The model under review builds one solid part; all positions refer to its coordinate system, in mm. Face numbers are marked on the shaded views. A direction names the side the tool comes from. Round coordinates to 2 decimals unless told otherwise and drop trailing zeros. Write each loop counter-clockwise with the first axis right and the second up, starting at its lowest first coordinate (ties: lowest second). Pieces come first, ordered by that corner, then holes. Notation, with made-up numbers: (-12.5, -3.75) - (22.5, -3.75) arc R25 ccw to (22.5, 31.25) - close; hole circle Ø1 at (40, -26). An arc over 180 degrees is marked (long way). Return JSON: item names as keys, results as strings.
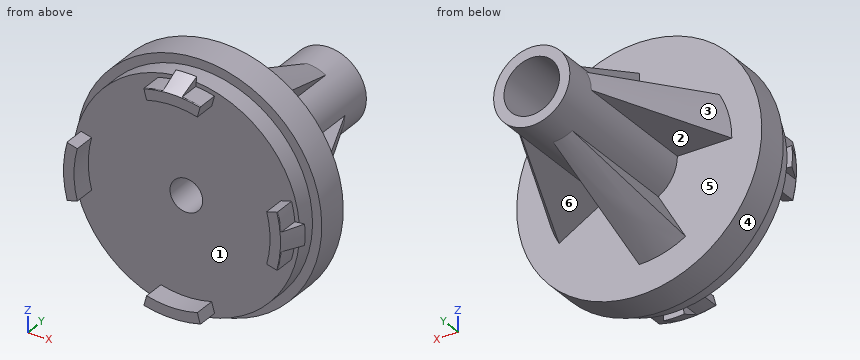
from build123d import *

# Parameters (mm, degrees)
SKETCH_1_R          = 10.4
EXTRUDE_1_DEPTH     = 1.8
SKETCH_2_R          = 11.25
EXTRUDE_2_DEPTH     = 3
SKETCH_3_R          = 3.5
SKETCH_3_R_2        = 2.55
EXTRUDE_3_DEPTH     = 15
SKETCH_3_4_R        = 1.5
CUT_EXTRUDE_2_DEPTH = 4.8
REVOLVE_3_ANGLE     = 30
REVOLVE_4_ANGLE     = 30
EXTRUDE_4_DEPTH     = 2


with BuildPart() as part:
    # 草图1 → 凸台-拉伸1 (new body)
    with BuildSketch(Plane(origin=(0, 0, 0), x_dir=(1, 0, 0), z_dir=(0, 1, 0))):
        with Locations(Location((0, 0, 0), (0, 0, 270))):
            Circle(SKETCH_1_R)
    extrude(amount=EXTRUDE_1_DEPTH)

    # 草图2 → 凸台-拉伸2 (add)
    with BuildSketch(Plane(origin=(0, 1.8, 0), x_dir=(1, 0, 0), z_dir=(0, 1, 0))):
        with Locations(Location((0, 0, 0), (0, 0, 270))):
            Circle(SKETCH_2_R)
    extrude(amount=EXTRUDE_2_DEPTH)

    # 草图3 → 凸台-拉伸3 (add)
    with BuildSketch(Plane(origin=(0, 4.8, 0), x_dir=(1, 0, 0), z_dir=(0, 1, 0))):
        with Locations(Location((0, 0, 0), (0, 0, 270))):
            Circle(SKETCH_3_R)
        with Locations(Location((0, 0, 0), (0, 0, 270))):
            Circle(SKETCH_3_R_2, mode=Mode.SUBTRACT)
    extrude(amount=EXTRUDE_3_DEPTH)

    # 草图3<4> → 切除-拉伸2 (cut)
    with BuildSketch(Plane(origin=(0, 4.8, 0), x_dir=(1, 0, 0), z_dir=(0, 1, 0))):
        with Locations(Location((0, 0, 0), (0, 0, 270))):
            Circle(SKETCH_3_4_R)
    extrude(amount=-CUT_EXTRUDE_2_DEPTH, mode=Mode.SUBTRACT)

    # 草图6 → 旋转3 (revolve)
    with BuildSketch(Plane(origin=(0, 0, 0), x_dir=(0, 0, -1), z_dir=(1, 0, 0))):
        Polygon((3.5, 4.8), (3.5, 16.8), (8.5, 4.8), align=None)
        Polygon((-8.5, 4.8), (-3.5, 4.8), (-3.5, 16.8), align=None)
    revolve(axis=Axis((0, 0, 0), (0, 1, 0)), revolution_arc=REVOLVE_3_ANGLE)

    # 草图9 → 旋转4 (revolve)
    with BuildSketch(Plane.XY):
        Polygon((3.5, 4.8), (8.5, 4.8), (3.5, 16.8), align=None)
        Polygon((-8.5, 4.8), (-3.5, 16.8), (-3.5, 4.8), align=None)
    revolve(axis=Axis((0, 0, 0), (0, 1, 0)), revolution_arc=REVOLVE_4_ANGLE)

    # 草图10 → 凸台-拉伸4 (add)
    with BuildSketch(Plane.XZ):
        with BuildLine():
            Line((9.961946981, -0.871557427), (10.858522209, -0.949997596))
            ThreePointArc((10.858522209, -0.949997596), (10.9, 0), (10.858522209, 0.949997596))
            Line((10.858522209, 0.949997596), (9.961946981, 0.871557427))
            ThreePointArc((9.961946981, 0.871557427), (9.84807753, 1.736481777), (9.659258263, 2.588190451))
            Line((9.659258263, 2.588190451), (8.693332437, 2.329371406))
            ThreePointArc((8.693332437, 2.329371406), (9, 0), (8.693332437, -2.329371406))
            Line((8.693332437, -2.329371406), (9.659258263, -2.588190451))
            ThreePointArc((9.659258263, -2.588190451), (9.84807753, -1.736481777), (9.961946981, -0.871557427))
        make_face()
        with BuildLine():
            Line((2.329371406, 8.693332437), (2.588190451, 9.659258263))
            ThreePointArc((2.588190451, 9.659258263), (1.736481777, 9.84807753), (0.871557427, 9.961946981))
            Line((0.871557427, 9.961946981), (0.949997596, 10.858522209))
            ThreePointArc((0.949997596, 10.858522209), (0, 10.9), (-0.949997596, 10.858522209))
            Line((-0.949997596, 10.858522209), (-0.871557427, 9.961946981))
            ThreePointArc((-0.871557427, 9.961946981), (-1.736481777, 9.84807753), (-2.588190451, 9.659258263))
            Line((-2.588190451, 9.659258263), (-2.329371406, 8.693332437))
            ThreePointArc((-2.329371406, 8.693332437), (0, 9), (2.329371406, 8.693332437))
        make_face()
        with BuildLine():
            Line((-2.329371406, -8.693332437), (-2.588190451, -9.659258263))
            ThreePointArc((-2.588190451, -9.659258263), (-1.736481777, -9.84807753), (-0.871557427, -9.961946981))
            Line((-0.871557427, -9.961946981), (-0.949997596, -10.858522209))
            ThreePointArc((-0.949997596, -10.858522209), (0, -10.9), (0.949997596, -10.858522209))
            Line((0.949997596, -10.858522209), (0.871557427, -9.961946981))
            ThreePointArc((0.871557427, -9.961946981), (1.736481777, -9.84807753), (2.588190451, -9.659258263))
            Line((2.588190451, -9.659258263), (2.329371406, -8.693332437))
            ThreePointArc((2.329371406, -8.693332437), (0, -9), (-2.329371406, -8.693332437))
        make_face()
        with BuildLine():
            Line((-8.693332437, 2.329371406), (-9.659258263, 2.588190451))
            ThreePointArc((-9.659258263, 2.588190451), (-9.84807753, 1.736481777), (-9.961946981, 0.871557427))
            Line((-9.961946981, 0.871557427), (-10.858522209, 0.949997596))
            ThreePointArc((-10.858522209, 0.949997596), (-10.9, 0), (-10.858522209, -0.949997596))
            Line((-10.858522209, -0.949997596), (-9.961946981, -0.871557427))
            ThreePointArc((-9.961946981, -0.871557427), (-9.84807753, -1.736481777), (-9.659258263, -2.588190451))
            Line((-9.659258263, -2.588190451), (-8.693332437, -2.329371406))
            ThreePointArc((-8.693332437, -2.329371406), (-9, 0), (-8.693332437, 2.329371406))
        make_face()
    extrude(amount=EXTRUDE_4_DEPTH)

    # 草图11 → 切除-旋转2 (revolve, cut)
    with BuildSketch(Plane.XY, mode=Mode.PRIVATE) as cut_revolve_2_sk:
        Polygon((9.961946981, -2), (10.9, -2), (10.9, 0), align=None)
    revolve(cut_revolve_2_sk.sketch.rotate(Axis((0, 0, 0), (0, -1, 0)), 275), axis=Axis((0, 0, 0), (0, -1, 0)), mode=Mode.SUBTRACT)


solid = part.part
(1) Add section A-A (y = 6.25). Write out the cut boundary in (x, z).
Filled in:
{"outline": "(-7.9, 0) - (-3.5, 0) arc R3.5 ccw to (-1.75, -3.03) - (-3.95, -6.84) arc R7.9 ccw to (0, -7.9) - (0, -3.5) arc R3.5 ccw to (3.03, -1.75) - (6.84, -3.95) arc R7.9 ccw to (7.9, 0) - (3.5, 0) arc R3.5 ccw to (1.75, 3.03) - (3.95, 6.84) arc R7.9 ccw to (0, 7.9) - (0, 3.5) arc R3.5 ccw to (-3.03, 1.75) - (-6.84, 3.95) arc R7.9 ccw to start; hole circle Ø5.1 at (0, 0)"}
(2) For the marked faces 4, 5 and 6, list the 3-axis set-ups (+Z, -Z, +X, -X, +Y, -Y) from which the entire face can be reached by the end or side of a thin tool; tool diameter is ignored.
Filled in:
{"face 4": "+Y, -Y", "face 5": "+Y", "face 6": "-Z, +Y"}
(3) Clearance check with flat-ended pins moving along their axes: pin 1 Ø4 at (x, z) = (-1, -0.5) entering from +Y; pin 2 Ø5.5 at (y, z) = (12, -7) entering from +X; pin 3 Ø1.5 at (y, z) = (8.5, 6.5) entering from -X; pin 4 Ø1 at (x, z) = (0.5, 7.5) entering from -Y. State where each tip first meets the part, or that it passes through.
Filled in:
{"pin 1": "stops at y = 19.8", "pin 2": "stops at x = 0", "pin 3": "stops at x = 0", "pin 4": "stops at y = 0"}
(4) Add section B-B (y = 14.5). Write out the cut boundary in (x, z), plus the area to 3 significant figures.
Filled in:
{"outline": "(-4.46, 0) - (-3.5, 0) arc R3.5 ccw to (-1.75, -3.03) - (-2.23, -3.86) arc R4.46 ccw to (0, -4.46) - (0, -3.5) arc R3.5 ccw to (3.03, -1.75) - (3.86, -2.23) arc R4.46 ccw to (4.46, 0) - (3.5, 0) arc R3.5 ccw to (1.75, 3.03) - (2.23, 3.86) arc R4.46 ccw to (0, 4.46) - (0, 3.5) arc R3.5 ccw to (-3.03, 1.75) - (-3.86, 2.23) arc R4.46 ccw to start; hole circle Ø5.1 at (0, 0)", "area": "26.0 mm2"}
(5) Mouldability with a two-part tool opening along X and no side actions: class the marked faces 1, 2 and 3 as released by +X, released by -X, zero draft, split by the parting line, or undercut.
Filled in:
{"face 1": "undercut", "face 2": "zero draft", "face 3": "released by -X"}
(6) Wall thickness on line 1 (Z direction, x = -2, y = 5); line 2 (X direction, y = 1.95, z = 0); line 3 (Y direction, x = 2.25, z = 1.75): over which ranges is each line inside the solid? List them lowest first.
Filled in:
{"line 1": "z = -8.18 to -3.46, -2.87 to -1.58, 1.58 to 2.87", "line 2": "x = -11.25 to -1.5, 1.5 to 11.25", "line 3": "y = 0 to 19.8"}
(7) Add section C-C (y = 3). Write out the cut boundary in (x, z).
Filled in:
{"outline": "circle Ø22.5 at (0, 0); hole circle Ø3 at (0, 0)"}
